Can you work these out from the model? Positions are in its coordinate system, mm. Face numbers are marked on the shaded views. A direction names the side the tool comes from. Coordinates: 2 decimals unless noted, no trailing zeros. Order: outer loops, then holes, each group sorted by start corner. A loop starts at its lowest first (then second) coordinate and runs counter-clockwise, first axis right, second up. Notation, with made-up numbers: (-3.75, 52.25) -> (18.25, 52.25) arc R10 cw to (18.25, 60.25) -> close; hole circle Ø8 at (81, 18). An arc over 180 degrees is marked (long way). Use a Markdown table: item, result. Add a question column.
1. Suppose I cut it at D-D, the plane z = -3. List the corners of the cut face in (x, y) for me.
2. Suppose I cut it at B-B, the plane y = 17. List the corners of the cut face in (x, z) for me, then the cut area to 3 significant figures.
3. Suppose I cut it at C-C, the plane x = -9.5. List the corners of the cut face in (y, z) for me, then the cut area to 3 significant figures.
4. For the marked faces 1, 2, 3, 4 and 5, which set-ups out of +Z, -Z, +X, -X, +Y, -Y let a thin tool reach every point of the face, with its end or its side?
5. For pin 1 Ø1.5 at (x, y) = (1, 1) entering from +Z; pin 2 Ø5 at (x, y) = (9.5, -11.5) entering from -Z; pin 3 Ø1 at (x, z) = (24, 14.5) entering from +Y, each with a flat end and sliding along its axis, tell me the tip position at first contact or that it passes through.
6. If I drill on line 1 along Y through (x, z) = (40, -4.5); line 2 along Z through (x, y) = (0, 6.75); line 3 along Z through (x, y) = (0, 19), over which ranges is the centre line in solid material (lowest first)? Write a range as from..to.
7. Suppose I cut it at A-A, the plane z = -9. List the corners of the cut face in (x, y) for me.
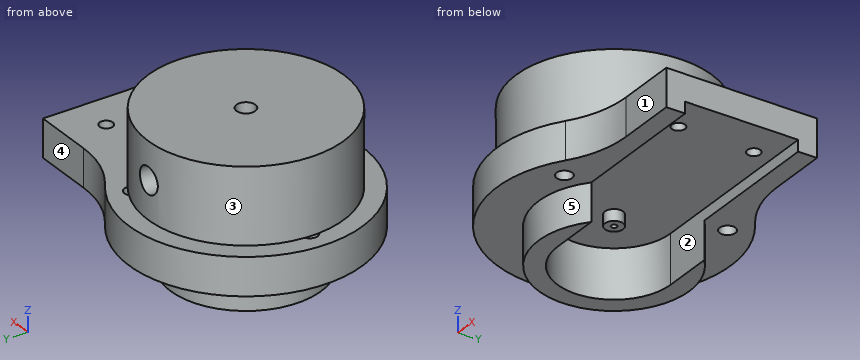
```python
from build123d import *

# Parameters (mm, degrees)
SKETCH1_R                     = 26
BOSS_EXTRUDE1_DEPTH           = 20
SKETCH2_W                     = 2.1
SKETCH2_H                     = 26
SKETCH4_R                     = 3.5
CUT_EXTRUDE1_DEPTH            = 15
BOSS_EXTRUDE2_DEPTH           = 10
CUT_EXTRUDE2_DEPTH            = 3
SKETCH7_R                     = 2.4
BOSS_EXTRUDE3_DEPTH           = 3
SKETCH8_R                     = 0.75
CUT_EXTRUDE3_DEPTH            = 67.03786797
SKETCH9_R                     = 2.5
CUT_EXTRUDE4_DEPTH            = 14
SKETCH10_R                    = 1.75
CUT_EXTRUDE5_DEPTH            = 16
BOSS_EXTRUDE4_START           = 10
BOSS_EXTRUDE4_DEPTH           = 10
M5X0_8_START                  = -10
M5X0_8_TAPPED_HOLE2_OUTLINE_R = 2.1
M5X0_8_TAPPED_HOLE2_DEPTH     = 10
CIRPATTERN1_COUNT             = 3


# Read off the part's stored shape, not the designer's step: M5x0.8 Tapped Hole2
with BuildPart() as part:
    # Sketch1 → Boss-Extrude1 (new body)
    with BuildSketch(Plane.XY):
        Circle(SKETCH1_R)
    extrude(amount=BOSS_EXTRUDE1_DEPTH)

    # Sketch2 → M5x0.8 Tapped Hole1 (revolve, cut)
    with BuildSketch(Plane(origin=(0, 0, 10), x_dir=(0, 0, -1), z_dir=(1, 0, 0))):
        with Locations((1.05, 13)):
            Rectangle(SKETCH2_W, SKETCH2_H)
    revolve(axis=Axis((0, -6.35, 10), (0, 1, 0)), mode=Mode.SUBTRACT)

    # Sketch4 → Cut-Extrude1 (cut)
    with BuildSketch(Plane(origin=(0, 26, 0), x_dir=(-1, 0, 0), z_dir=(0, 1, 0))):
        with Locations(Location((0, 10, 0), (0, 0, 90))):
            Circle(SKETCH4_R)
    extrude(amount=-CUT_EXTRUDE1_DEPTH, mode=Mode.SUBTRACT)

    # Sketch5 → Boss-Extrude2 (add)
    with BuildSketch(Plane(origin=(0, 0, 0), x_dir=(-1, 0, 0), z_dir=(0, 0, -1))):
        with BuildLine():
            Line((-34.142470626, -20), (-50, -20))
            Line((-50, -20), (-50, 20))
            Line((-50, 20), (-34.142470626, 20))
            ThreePointArc((-34.142470626, 20), (-25.713473942, 21.324307139), (-18.096692901, 25.16961871))
            ThreePointArc((-18.096692901, 25.16961871), (31, 0), (-18.096692901, -25.16961871))
            ThreePointArc((-18.096692901, -25.16961871), (-25.713473942, -21.324307139), (-34.142470626, -20))
        make_face()
    extrude(amount=BOSS_EXTRUDE2_DEPTH)

    # Sketch6 → Cut-Extrude2 (cut)
    with BuildSketch(Plane(origin=(0, 0, -10), x_dir=(-1, 0, 0), z_dir=(0, 0, -1))):
        with BuildLine():
            Line((0, -15), (-80, -15))
            ThreePointArc((-80, -15), (-95, 0), (-80, 15))
            Line((-80, 15), (0, 15))
            ThreePointArc((0, 15), (15, 0), (0, -15))
        make_face()
    extrude(amount=-CUT_EXTRUDE2_DEPTH, mode=Mode.SUBTRACT)

    # Sketch7 → Boss-Extrude3 (add)
    with BuildSketch(Plane(origin=(0, 0, -7), x_dir=(-1, 0, 0), z_dir=(0, 0, -1))):
        with Locations(Location((0, 0, 0), (0, 0, 180))):
            Circle(SKETCH7_R)
    extrude(amount=BOSS_EXTRUDE3_DEPTH)

    # Sketch8 → Cut-Extrude3 (cut, through all)
    with BuildSketch(Plane(origin=(0, 0, -10), x_dir=(-1, 0, 0), z_dir=(0, 0, -1))):
        Circle(SKETCH8_R)
    extrude(amount=-CUT_EXTRUDE3_DEPTH, mode=Mode.SUBTRACT)

    # Sketch9 → Cut-Extrude4 (cut)
    with BuildSketch(Plane.XY.offset(20)):
        Circle(SKETCH9_R)
    extrude(amount=-CUT_EXTRUDE4_DEPTH, mode=Mode.SUBTRACT)

    # Sketch10 → Cut-Extrude5 (cut)
    with BuildSketch(Plane(origin=(0, 0, -7), x_dir=(-1, 0, 0), z_dir=(0, 0, -1))):
        with Locations((-40, -10)):
            Circle(SKETCH10_R)
        with Locations((-40, 10)):
            Circle(SKETCH10_R)
    extrude(amount=-CUT_EXTRUDE5_DEPTH, mode=Mode.SUBTRACT)

    # Sketch11 → Boss-Extrude4 (add)
    with BuildSketch(Plane(origin=(0, 0, -10), x_dir=(-1, 0, 0), z_dir=(0, 0, -1)).offset(BOSS_EXTRUDE4_START)):
        with BuildLine():
            Line((0, 15), (-13.228756555, 15))
            ThreePointArc((-13.228756555, 15), (20, 0), (-13.228756555, -15))
            Line((-13.228756555, -15), (0, -15))
            ThreePointArc((0, -15), (15, 0), (0, 15))
        make_face()
    extrude(amount=-BOSS_EXTRUDE4_DEPTH)

    # M5x0.8 Tapped Hole2 outline → M5x0.8 Tapped Hole2 (cut)
    with BuildSketch(Plane.XY.offset(M5X0_8_START)):
        with Locations((-25, 0)):
            Circle(M5X0_8_TAPPED_HOLE2_OUTLINE_R)
    m5x0_8_tapped_hole2 = extrude(amount=M5X0_8_TAPPED_HOLE2_DEPTH, mode=Mode.SUBTRACT)

    # CirPattern1: M5x0.8 Tapped Hole2 ×3 about axis
    cirpattern1_axis = Axis((0, 0, 0), (0, 0, 1))
    for i in range(1, CIRPATTERN1_COUNT):
        add(m5x0_8_tapped_hole2.rotate(cirpattern1_axis, i * 360 / CIRPATTERN1_COUNT), mode=Mode.SUBTRACT)


solid = part.part
```
Worked out:
| question | item | result |
|---|---|---|
| 1 | outline | (18.1, -25.17) arc R27.49 cw to (34.14, -20) -> (50, -20) -> (50, 20) -> (34.14, 20) arc R27.49 cw to (18.1, 25.17) arc R31 ccw (long way) to start; hole circle Ø4.2 at (-25, 0); hole circle Ø1.5 at (0, 0); hole circle Ø4.2 at (12.5, -21.65); hole circle Ø4.2 at (12.5, 21.65); hole circle Ø3.5 at (40, -10); hole circle Ø3.5 at (40, 10) |
| 2 | outline | (-25.92, -10) -> (-10.54, -10) -> (-10.54, -20) -> (10.54, -20) -> (10.54, -10) -> (50, -10) -> (50, 0) -> (19.67, 0) -> (19.67, 20) -> (-19.67, 20) -> (-19.67, 0) -> (-25.92, 0) -> close; hole circle Ø7 at (0, 10) |
| 2 | area | 1,720 mm² |
| 3 | outline | (-29.51, -10) -> (-17.6, -10) -> (-17.6, -20) -> (-11.61, -20) -> (-11.61, -7) -> (11.61, -7) -> (11.61, -20) -> (17.6, -20) -> (17.6, -10) -> (29.51, -10) -> (29.51, 0) -> (24.2, 0) -> (24.2, 20) -> (-24.2, 20) -> (-24.2, 0) -> (-29.51, 0) -> close |
| 3 | area | 1,610 mm² |
| 4 | face 1 | +Z, -Z, +X, -Y |
| 4 | face 2 | -Z, +X |
| 4 | face 3 | +Z |
| 4 | face 4 | +Z, -Z, +X, +Y |
| 4 | face 5 | -Z |
| 5 | pin 1 | stops at z = 6 |
| 5 | pin 2 | stops at z = -7 |
| 5 | pin 3 | stops at y = 11.12 |
| 6 | line 1 | y = -20..-11.75, -8.25..8.25, 11.75..20 |
| 6 | line 2 | z = -7..7.9, 12.1..20 |
| 6 | line 3 | z = -20..6.5, 13.5..20 |
| 7 | outline | circle Ø4.8 at (0, 0); (0, -15) arc R15 cw to (0, 15) -> (50, 15) -> (50, 20) -> (34.14, 20) arc R27.49 cw to (18.1, 25.17) arc R31 ccw (long way) to (18.1, -25.17) arc R27.49 cw to (34.14, -20) -> (50, -20) -> (50, -15) -> close; hole circle Ø4.2 at (-25, 0); hole circle Ø1.5 at (0, 0); hole circle Ø4.2 at (12.5, -21.65); hole circle Ø4.2 at (12.5, 21.65) |
